Read the model definition and answer for the solid it produces. Units are mm, in the model's axes. Face numbers are marked on the shaded views. A direction names the side the tool comes from. Round coordinates to 2 decimals unless told otherwise and drop trailing zeros. Order: outer loops, then holes, each group sorted by start corner. A loop starts at its lowest first (then second) coordinate and runs counter-clockwise, first axis right, second up.
from build123d import *

# Parameters (mm, degrees)
SKETCH_1_W          = 16
SKETCH_1_H          = 10
EXTRUDE_1_DEPTH     = 3
SKETCH_2_W          = 3
SKETCH_2_H          = 10
EXTRUDE_2_DEPTH     = 8
SKETCH_3_R          = 1.5
CUT_EXTRUDE_1_DEPTH = 3
SKETCH_5_R          = 3
CUT_EXTRUDE_3_DEPTH = 2
SKETCH_7_W          = 0.4
SKETCH_7_H          = 10
CUT_EXTRUDE_4_DEPTH = 22
SKETCH_8_R          = 2.1
CUT_EXTRUDE_5_DEPTH = 4.2
SKETCH_9_W          = 8
SKETCH_9_H          = 10
EXTRUDE_3_DEPTH     = 2
SKETCH_10_W         = 11
SKETCH_10_H         = 10
CUT_EXTRUDE_6_DEPTH = 2
FILLET_1_R          = 0.4


with BuildPart() as part:
    # 草图1 → 凸台-拉伸1 (new body)
    with BuildSketch(Plane(origin=(0, 0, 0), x_dir=(0, 0, -1), z_dir=(1, 0, 0))):
        with Locations((-8, 5)):
            Rectangle(SKETCH_1_W, SKETCH_1_H)
    extrude(amount=EXTRUDE_1_DEPTH)

    # 草图2 → 凸台-拉伸2 (add)
    with BuildSketch(Plane(origin=(3, 0, 0), x_dir=(0, 0, -1), z_dir=(1, 0, 0))):
        with Locations((-1.9, 5)):
            Rectangle(SKETCH_2_W, SKETCH_2_H)
    extrude(amount=EXTRUDE_2_DEPTH)

    # 草图3 → 切除-拉伸1 (cut)
    with BuildSketch(Plane(origin=(3, 0, 0), x_dir=(0, 0, -1), z_dir=(1, 0, 0))):
        with Locations((-10, 5)):
            Circle(SKETCH_3_R)
    extrude(amount=-CUT_EXTRUDE_1_DEPTH, mode=Mode.SUBTRACT)

    # 草图5 → 切除-拉伸3 (cut)
    with BuildSketch(Plane(origin=(3, 0, 0), x_dir=(0, 0, -1), z_dir=(1, 0, 0))):
        with Locations((-10, 5)):
            Circle(SKETCH_5_R)
    extrude(amount=-CUT_EXTRUDE_3_DEPTH, mode=Mode.SUBTRACT)

    # 草图7 → 切除-拉伸4 (cut)
    with BuildSketch(Plane(origin=(3, 0, 0), x_dir=(0, 0, -1), z_dir=(1, 0, 0))):
        with Locations((-0.2, 5)):
            Rectangle(SKETCH_7_W, SKETCH_7_H)
    extrude(amount=-CUT_EXTRUDE_4_DEPTH, mode=Mode.SUBTRACT)

    # 草图8 → 切除-拉伸5 (cut)
    with BuildSketch(Plane(origin=(0, 0, 0.4), x_dir=(-1, 0, 0), z_dir=(0, 0, -1))):
        with Locations(Location((-7.8, 5, 0), (0, 0, 90))):
            Circle(SKETCH_8_R)
    extrude(amount=-CUT_EXTRUDE_5_DEPTH, mode=Mode.SUBTRACT)

    # 草图9 → 凸台-拉伸3 (add)
    with BuildSketch(Plane.XY.offset(3.4)):
        with Locations((7, 5)):
            Rectangle(SKETCH_9_W, SKETCH_9_H)
    extrude(amount=EXTRUDE_3_DEPTH)

    # 草图10 → 切除-拉伸6 (cut)
    with BuildSketch(Plane(origin=(0, 0, 0.4), x_dir=(-1, 0, 0), z_dir=(0, 0, -1))):
        with Locations((-5.5, 5)):
            Rectangle(SKETCH_10_W, SKETCH_10_H)
    extrude(amount=-CUT_EXTRUDE_6_DEPTH, mode=Mode.SUBTRACT)

    # 圆角1
    fillet_1_edges = [part.edges().sort_by_distance(p)[0] for p in [
        (7.8, 2.9, 2.4),
    ]]
    fillet(fillet_1_edges, radius=FILLET_1_R)


solid = part.part
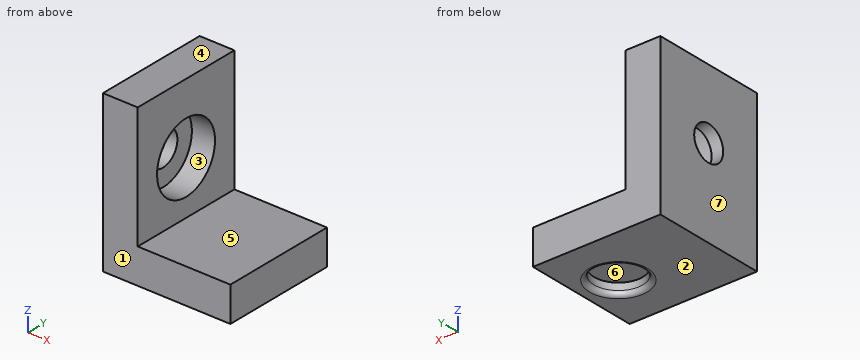
Q1. Straight lines are drawn through the part: probe 1 along Y at (x, z) = (2, 10); probe 2 along Z at (x, y) = (4.75, 3.75); probe 3 along X at (y, z) = (5, 3). For each, find the intervals that lie inside material, in ascending order.
Outcome:
probe 1: y = 0 to 2, 8 to 10
probe 2: z = 2.4 to 5.4
probe 3: x = 0 to 5.7, 9.9 to 11
Q2. For a pull along Z with two mould halves and no side action, classify the marked faces 1, 2, 3 and 4 as released by +Z, released by -Z, zero draft, split by the parting line, or undercut.
Outcome:
face 1: zero draft
face 2: released by -Z
face 3: undercut
face 4: released by +Z
Q3. A cutting plane is placed at D-D, the plane z = 13.25. Give the vertices of the cut face in (x, y), plus the area to 3 significant figures.
Outcome:
outline: (0, 0) - (3, 0) - (3, 10) - (0, 10) - close
area: 30.0 mm2
Q4. A cutting plane is placed at C-C, the plane y = 8.75. Give the vertices of the cut face in (x, z).
Outcome:
outline: (0, 2.4) - (11, 2.4) - (11, 5.4) - (3, 5.4) - (3, 16) - (0, 16) - close
Q5. A cutting plane is placed at A-A, the plane z = 10. Give the vertices of the cut face in (x, y), plus the area to 3 significant figures.
Outcome:
outline: (0, 0) - (3, 0) - (3, 2) - (1, 2) - (1, 3.5) - (0, 3.5) - close; (0, 6.5) - (1, 6.5) - (1, 8) - (3, 8) - (3, 10) - (0, 10) - close
area: 15.0 mm2
Q6. Flat-ended cylindrical pins translate along their axes: pin 1 (6 mm diameter, centred on y = 6.5, z = 11, fed in from +X); pin 2 (2.5 mm diameter, centred on x = 7.8, y = 5, fed in from -Z); pin 3 (5.5 mm diameter, centred on y = 5, z = 10, fed in from +X). Find the tip coordinate at first contact, or state that the pin passes through.
Outcome:
pin 1: stops at x = 3
pin 2: stops at z = 3.4
pin 3: stops at x = 1
Q7. A cutting plane is placed at B-B, the plane x = 7.8. Give the vertices of the cut face in (y, z), plus the area to 3 significant figures.
Outcome:
outline: (0, 2.4) - (2.5, 2.4) arc R0.4 ccw to (2.9, 2.8) - (2.9, 3.4) - (7.1, 3.4) - (7.1, 2.8) arc R0.4 ccw to (7.5, 2.4) - (10, 2.4) - (10, 5.4) - (0, 5.4) - close
area: 25.7 mm2
Q8. For the marked faces 5, 6 and 7, determine the directions among +Z, -Z, +X, -X, +Y, -Y from which every point of the face is accessible in a straight line to the end or side of a thin tool.
Outcome:
face 5: +Z, +X, +Y, -Y
face 6: -Z
face 7: +Z, -Z, -X, +Y, -Y
